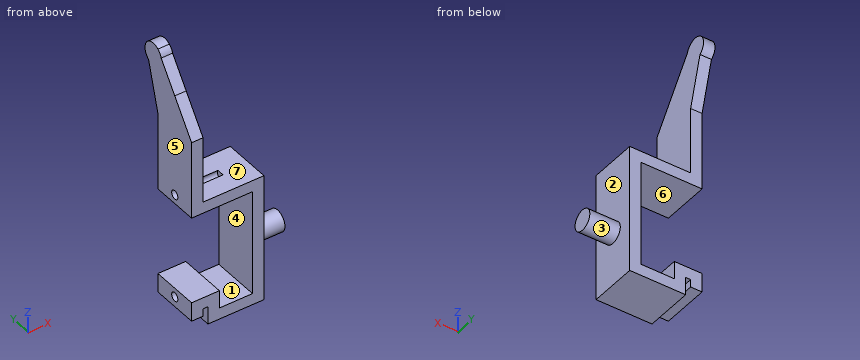
from build123d import *

# Parameters (mm, degrees)
EXTRUDE_1_DEPTH     = 12.5
SKETCH_2_R          = 1.15
CUT_EXTRUDE_1_DEPTH = 12
SKETCH_3_R          = 2.75
EXTRUDE_2_DEPTH     = 8
EXTRUDE_3_DEPTH     = 3
CUT_EXTRUDE_5_DEPTH = 3


with BuildPart() as part:
    # Sketch 1 → Extrude 1 (new body)
    with BuildSketch(Plane(origin=(0, 0, 0), x_dir=(1, 0, 0), z_dir=(0, 1, 0))):
        Polygon((0, 5), (0, 0), (7.3, 0), (7.3, 3), (7.3, 4.7), (16, 4.7), (16, 3), (16, 0), (16, -23), (0, -23), (0, -61), (3, -61), (3, -26), (19, -26), (19, 3), (19, 7.7), (4.3, 7.7), (4.3, 3), (3, 3), (3, 5), align=None)
    extrude(amount=EXTRUDE_1_DEPTH)

    # Sketch 2 → Cut-Extrude 1 (cut)
    with BuildSketch(Plane.ZY):
        with Locations((-2.35, 6.25)):
            Circle(SKETCH_2_R)
        with Locations((25.35, 6.25)):
            Circle(SKETCH_2_R)
    extrude(amount=-CUT_EXTRUDE_1_DEPTH, mode=Mode.SUBTRACT)

    # Sketch 3 → Extrude 2 (add)
    with BuildSketch(Plane(origin=(19, 0, 0), x_dir=(0, 0, -1), z_dir=(1, 0, 0))):
        with Locations((-6.35, 6.25)):
            Circle(SKETCH_3_R)
    extrude(amount=EXTRUDE_2_DEPTH)

    # Sketch 4 → Extrude 3 (add)
    with BuildSketch(Plane(origin=(3, 0, 0), x_dir=(0, 0, -1), z_dir=(1, 0, 0))):
        with BuildLine():
            Line((-61, 12.5), (-55.974372634, 12.5))
            ThreePointArc((-55.974372634, 12.5), (-55.572277982, 13.325961613), (-55.434075858, 14.234142689))
            ThreePointArc((-55.434075858, 14.234142689), (-55.572277982, 15.142323766), (-55.974372634, 15.968285379))
            ThreePointArc((-55.974372634, 15.968285379), (-60.221329006, 16.746956372), (-61, 12.5))
        make_face()
        with BuildLine():
            Line((-55.974372634, 12.5), (-43.5, 12.5))
            Line((-43.5, 12.5), (-55.974372634, 15.968285379))
            ThreePointArc((-55.974372634, 15.968285379), (-55.572277982, 15.142323766), (-55.434075858, 14.234142689))
            ThreePointArc((-55.434075858, 14.234142689), (-55.572277982, 13.325961613), (-55.974372634, 12.5))
        make_face()
    extrude(amount=-EXTRUDE_3_DEPTH)

    # Sketch 4_8 → Cut-Extrude 5 (cut)
    with BuildSketch(Plane(origin=(3, 0, 0), x_dir=(0, 0, -1), z_dir=(1, 0, 0))):
        with BuildLine():
            Line((-43.5, 0), (-52.25, 6.25))
            Line((-52.25, 6.25), (-59.312624964, 11.294732117))
            ThreePointArc((-59.312624964, 11.294732117), (-60.261770725, 11.749724518), (-61, 12.5))
            Line((-61, 12.5), (-61, 0))
            Line((-61, 0), (-43.5, 0))
        make_face()
    extrude(amount=-CUT_EXTRUDE_5_DEPTH, mode=Mode.SUBTRACT)


solid = part.part
Part model, mm, in its own coordinate system. Face numbers are marked on the shaded views. A direction names the side the tool comes from. Give positions to 0.01 mm unless a question says otherwise; leave off trailing zeros. Order: outer loops, then holes, each group sorted by start corner. A loop starts at its lowest first (then second) coordinate and runs counter-clockwise, first axis right, second up. Notation, with made-up numbers: (80, -40) -> (118, -40) arc R21 cw to (118, -27) -> close; hole circle Ø5 at (73, 37.25). An arc over 180 degrees is marked (long way). Use one line per item in the form item = value.
(1) Pull direction Z, two halves, no side cores. Call the marked faces 1, 2, 3 and 4: +Z half, -Z half, draft (parallel to the pull), parting line (faces both ways), or undercut.
Solution:
face_1 = undercut
face_2 = draft
face_3 = parting line
face_4 = undercut
(2) Saw through at C-C (z = 6.35). Write the cut outline in (x, y).
Solution:
outline = (16, 0) -> (19, 0) -> (19, 3.5) -> (27, 3.5) -> (27, 9) -> (19, 9) -> (19, 12.5) -> (16, 12.5) -> close
(3) Saw through at B-B (y = 1.5). Write the cut outline in (x, z).
Solution:
outline = (0, -5) -> (3, -5) -> (3, -3) -> (4.3, -3) -> (4.3, -7.7) -> (19, -7.7) -> (19, 26) -> (3, 26) -> (3, 45.6) -> (0, 45.6) -> (0, 23) -> (16, 23) -> (16, -4.7) -> (7.3, -4.7) -> (7.3, 0) -> (0, 0) -> close
(4) Flat gauge pins, fed straight in: P1, Ø6, axis at y = 11, z = 4, coming from the -X side; P2, Ø8, axis at y = 9, z = 25.5, coming from the +X side; P3, Ø2.5, axis at x = 1.5, y = 8.5, coming from the -Z side; P4, Ø2, axis at x = 13.5, z = 13.5, coming from the +Y side. Where does each tip first touch, or does it go through?
Solution:
P1 = 16
P2 = 19
P3 = -5
P4 = through
(5) Drill centre lines: line 1 (Z direction, x = 2.5, y = 6.25); line 2 (Z direction, x = 5, y = 7.5); line 3 (Z direction, x = 13.5, y = 1). Where is each one in solid material? Low to high. Write a range as from..to.
Solution:
line_1 = -5..-3.5, -1.2..0, 23..24.2, 26.5..52.25
line_2 = -7.7..0, 23..26
line_3 = -7.7..-4.7, 23..26
(6) Tool access for the marked faces 5, 6 and 7: list every direction of +Z, -Z, +X, -X, +Y, -Y with a clear straight run to the whole face (end or side of a thin tool).
Solution:
face_5 = +Z, -Z, -X, +Y, -Y
face_6 = -X, +Y, -Y
face_7 = +Z, +X, +Y, -Y
(7) Saw through at A-A (z = -2.35). Write the cut outline in (x, y).
Solution:
outline = (0, 0) -> (7.3, 0) -> (7.3, 5.1) -> (0, 5.1) -> close; (0, 7.4) -> (7.3, 7.4) -> (7.3, 12.5) -> (0, 12.5) -> close; (16, 0) -> (19, 0) -> (19, 12.5) -> (16, 12.5) -> close
(8) Saw through at D-D (x = 17.5). Write the cut outline in (y, z), then the cut area to 3 significant figures.
Solution:
outline = (0, -7.7) -> (12.5, -7.7) -> (12.5, 26) -> (0, 26) -> close
area = 421 mm²
